Input: part model. Units: mm. Frame: model coordinates. Face numbers are marked on the shaded views. Coordinates: 2 decimals unless noted, no trailing zeros. Loops run counter-clockwise (first coordinate to the right, second up) from the corner with the lowest first, then second, coordinate; pieces in that order, holes last. Notation, with made-up numbers: M 22,26 L 62,26 A7 cw 62,37 Z; hole C 15,52.25 d9. An arc over 180 degrees is marked long. Use a Markdown table: item, result. Add a question column.
1. Line query: L1, parallel to Z at x = -7.5, y = 8.25; L2, parallel to X at y = 0.5, z = 76; L3, parallel to X at y = 9.25, z = 48. Output: solid intervals per line, ascending. Write a range as [from, to].
2. Section A-A on x = 0. Output: boundary loops of the cut face in (y, z).
3. Pin query (flat end, axial travel): pin 1 (6 mm diameter, centred on y = 4.5, z = 71.5, fed in from -X); pin 2 (2 mm diameter, centred on x = 8.5, z = 10, fed in from +Y); pin 3 (10 mm diameter, centred on x = -1.5, z = 72, fed in from +Y); pin 4 (1.5 mm diameter, centred on y = 8, z = 62.5, fed in from -X). Return the tip coordinate at first contact, or that it passes through.
4. Draft query along Z for the marked faces 1, 2 and 3. Return one class per face: +Z half, -Z half, draft (parallel to the pull), parting line (faces both ways), or undercut.
5. Section D-D on z = 15. Output: boundary loops of the cut face in (x, y), then the cut area to 3 significant figures.
6. Section C-C on y = 11.5. Output: boundary loops of the cut face in (x, z).
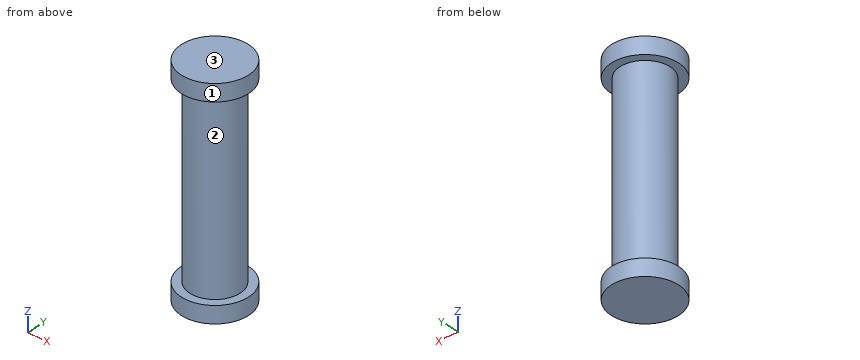
```python
from build123d import *

# Parameters (mm, degrees)
SKETCH_1_R      = 30
EXTRUDE_1_DEPTH = 220
SKETCH_2_R      = 40
EXTRUDE_2_DEPTH = 20
EXTRUDE_START   = 20
SKETCH_3_R      = 40
EXTRUDE_3_DEPTH = 20
SCALE_1_SCALE   = 0.345


with BuildPart() as part:
    # 草图1 → 凸台-拉伸1 (new body)
    with BuildSketch(Plane.XY):
        Circle(SKETCH_1_R)
    extrude(amount=EXTRUDE_1_DEPTH)

    # 草图2 → 凸台-拉伸2 (add)
    with BuildSketch(Plane.XY.offset(220)):
        Circle(SKETCH_2_R)
    extrude(amount=EXTRUDE_2_DEPTH)

    # 草图3 → 凸台-拉伸3 (add)
    with BuildSketch(Plane(origin=(0, 0, 0), x_dir=(-1, 0, 0), z_dir=(0, 0, -1)).offset(EXTRUDE_START)):
        with Locations(Location((0, 0, 0), (0, 0, 180))):
            Circle(SKETCH_3_R)
    extrude(amount=-EXTRUDE_3_DEPTH)


with BuildPart() as part_1:
    # 缩放比例1: scaled about (0, 0, 0)
    add(part.part.scale(SCALE_1_SCALE))


solid = part_1.part
```
Answers below:
| question | item | result |
|---|---|---|
| 1 | L1 | z = [-6.9, 0], [75.9, 82.8] |
| 1 | L2 | x = [-13.79, 13.79] |
| 1 | L3 | x = [-4.64, 4.64] |
| 2 | outline | M -13.8,-6.9 L 13.8,-6.9 L 13.8,0 L 10.35,0 L 10.35,75.9 L 13.8,75.9 L 13.8,82.8 L -13.8,82.8 L -13.8,75.9 L -10.35,75.9 L -10.35,0 L -13.8,0 Z |
| 3 | pin 1 | stops at x = -10.24 |
| 3 | pin 2 | stops at y = 7.13 |
| 3 | pin 3 | stops at y = 13.8 |
| 3 | pin 4 | stops at x = -7.39 |
| 4 | face 1 | draft |
| 4 | face 2 | undercut |
| 4 | face 3 | +Z half |
| 5 | outline | C 0,0 d20.7 |
| 5 | area | 337 mm² |
| 6 | outline | M -7.63,-6.9 L 7.63,-6.9 L 7.63,0 L -7.63,0 Z; M -7.63,75.9 L 7.63,75.9 L 7.63,82.8 L -7.63,82.8 Z |
